Part model, mm, in its own coordinate system. A direction names the side the tool comes from. Round coordinates to 2 decimals unless told otherwise and drop trailing zeros. Loops run counter-clockwise (first coordinate to the right, second up) from the corner with the lowest first, then second, coordinate; pieces in that order, holes last.
(1) Probe probe 1 along Z at (x, y) = (-15.5, 654.5); probe 2 along Z at (x, y) = (-19, 479); probe 3 along Y at (x, z) = (-18, -9). List the from-to ranges inside material, lowest first.
(2) Tool access for faces 4 (the face through (2, 345, 36)), 5 (the face through (0, 345, -40)): list every direction of +Z, -Z, +X, -X, +Y, -Y with a clear straight run to the whole face (end or side of a thin tool).
(3) Cut at B-B on y = 625. List the corners of the cut face in (x, z).
(4) Flat gauge pins, fed straight in: pin 1 (1 mm diameter, centred on y = 108.5, z = 7.5, fed in from +X); pin 2 (10.5 mm diameter, centred on y = 479, z = -27.5, fed in from -X). Where does each tip first touch, or does it go through?
(5) Mould opens along Z. For faces 1 (the face through (0, 345, 40)), 2 (the face through (-16.4, 3.6, 0.2)), 3 (the face through (-16, 345, 1)) say: +Z half, -Z half, draft (parallel to the pull), parting line (faces both ways), or undercut.
(6) Cut at C-C on z = 29. List the corners of the cut face in (x, y), then the cut area to 3 significant figures.
(7) Cut at A-A on x = -4.5. List the corners of the cut face in (y, z).
Solid Edge part; units mm, degrees
sketch "Sketch1" plane through (0, 0, 0) normal (0, -1, 0) x (1, 0, 0)
  line L0 (20, 36) -> (-16, 36)
  line L1 (-16, 36) -> (-16, -36)
  line L2 (-16, -36) -> (20, -36)
  line L3 (20, -36) -> (20, -40)
  line L4 (20, -40) -> (-20, -40)
  line L5 (-20, -40) -> (-20, 40)
  line L6 (-20, 40) -> (20, 40)
  line L7 (20, 40) -> (20, 36)
  dimension "D1" = 20
  dimension "D2" = 20
  dimension "D3" = 20
extrude "Protrusion1" add sketch "Sketch1" against normal blind 700
sketch "Sketch2" plane through (0, 350, 40) normal (0, 0, 1) x (0, 1, 0)
  line L0 (-350, 20) -> (-310, -20)
extrude "Cutout1" cut sketch "Sketch2" against normal through all material side at (0.0354, 19.9646, 40)
sketch "Sketch3" plane through (0, 350, 40) normal (0, 0, 1) x (0, 1, 0)
  line L0 (350, 20) -> (310, -20)
extrude "Cutout2" cut sketch "Sketch3" against normal through all material side at (0.0354, 680.0354, 40)
sketch "Sketch4" plane through (-16, 350, 0) normal (1, 0, 0) x (0, 1, 0)
  circle A0 centre (-126, 10) radius 3.3
  circle A1 centre (34, 10) radius 3.3
extrude "Cutout3" cut sketch "Sketch4" against normal through all
hole "Bohrung_1" at (-16, 591, -9.5) direction (-1, 0, 0) diameter 6.6 end up to next
hole "Hole1" at (-16, 565, -27.5) direction (-1, 0, 0) diameter 6.6 end up to next
hole "Hole2" at (-16, 453, -9.5) direction (-1, 0, 0) diameter 6.6 end up to next
hole "Hole3" at (-16, 479, -27.5) direction (-1, 0, 0) diameter 6.6 end up to next
Final values:
1. probe 1: z = -40 to -36, 36 to 40
1. probe 2: z = -40 to -30.8, -24.2 to 40
1. probe 3: y = 2 to 449.74, 456.26 to 587.74, 594.26 to 698
2. face 4: +X, +Y, -Y
2. face 5: -Z, +X, -X, +Y, -Y
3. outline: (-20, -40) - (20, -40) - (20, -36) - (-16, -36) - (-16, 36) - (20, 36) - (20, 40) - (-20, 40) - close
4. pin 1: stops at x = -16
4. pin 2: stops at x = -20
5. face 1: +Z half
5. face 2: draft
5. face 3: undercut
6. outline: (-20, 0) - (-16, 4) - (-16, 696) - (-20, 700) - close
6. area: 2,780 mm2
7. outline: (15.5, -40) - (684.5, -40) - (684.5, -36) - (15.5, -36) - close; (15.5, 36) - (684.5, 36) - (684.5, 40) - (15.5, 40) - close
